from build123d import *

# Parameters (mm, degrees)
BOSS_EXTRUDE1_DEPTH      = 2
BOSS_EXTRUDE1_DEPTH_BACK = 1.043576075
SKETCH1_W                = 32
SKETCH1_H                = 40
CUT_EXTRUDE3_DEPTH       = 26.792699652
CUT_EXTRUDE3_DEPTH_BACK  = 26.792699652
SKETCH5_R                = 1.5
SKETCH5_R_2              = 1
SKETCH_4_W               = 14
SKETCH_4_H               = 4.843949414
CUT_EXTRUDE_3_DEPTH      = 26.792699652
SKETCH_5_W               = 9
SKETCH_5_H               = 3
EXTRUDE_3_DEPTH          = 10
SKETCH_6_R               = 1.5
CUT_EXTRUDE_5_DEPTH      = 44.8178046


with BuildPart() as part:
    # Sketch1 → Boss-Extrude1 (new, two sides: drawn at the far end of the back side and taken through both)
    with BuildSketch(Plane.XY.offset(-BOSS_EXTRUDE1_DEPTH_BACK)):
        Rectangle(SKETCH1_W, SKETCH1_H)
    extrude(amount=BOSS_EXTRUDE1_DEPTH + BOSS_EXTRUDE1_DEPTH_BACK)

    # Sketch5 → Cut-Extrude3 (cut, two sides: drawn at the far end of the back side and taken through both)
    with BuildSketch(Plane.XY.offset(2).offset(-CUT_EXTRUDE3_DEPTH_BACK)):
        Circle(SKETCH5_R)
        with Locations((0, 7.2)):
            Circle(SKETCH5_R_2)
        with Locations((7.2, 0)):
            Circle(SKETCH5_R_2)
        with Locations((0, -7.2)):
            Circle(SKETCH5_R_2)
        with Locations((-7.2, 0)):
            Circle(SKETCH5_R_2)
    extrude(amount=CUT_EXTRUDE3_DEPTH + CUT_EXTRUDE3_DEPTH_BACK, mode=Mode.SUBTRACT)

    # 草图4 → 切除-拉伸3 (cut, through all)
    with BuildSketch(Plane.XY.offset(2)):
        with Locations((0, 17.578025293)):
            Rectangle(SKETCH_4_W, SKETCH_4_H)
        with Locations((0, -17.578025293)):
            Rectangle(SKETCH_4_W, SKETCH_4_H)
    extrude(amount=-CUT_EXTRUDE_3_DEPTH, mode=Mode.SUBTRACT)

    # 草图5 → 凸台-拉伸3 (add)
    with BuildSketch(Plane.XY.offset(2)):
        with Locations((11.5, 18.5)):
            Rectangle(SKETCH_5_W, SKETCH_5_H)
        with Locations((-11.5, 18.5)):
            Rectangle(SKETCH_5_W, SKETCH_5_H)
        with Locations((-11.5, -18.5)):
            Rectangle(SKETCH_5_W, SKETCH_5_H)
        with Locations((11.5, -18.5)):
            Rectangle(SKETCH_5_W, SKETCH_5_H)
    extrude(amount=-EXTRUDE_3_DEPTH)

    # 草图6 → 切除-拉伸5 (cut, through all)
    with BuildSketch(Plane.XZ.offset(20)):
        with Locations(Location((11.6894988, -5, 0), (0, 0, 270))):
            Circle(SKETCH_6_R)
        with Locations(Location((-11.6894988, -5, 0), (0, 0, 270))):
            Circle(SKETCH_6_R)
    extrude(amount=-CUT_EXTRUDE_5_DEPTH, mode=Mode.SUBTRACT)


solid = part.part
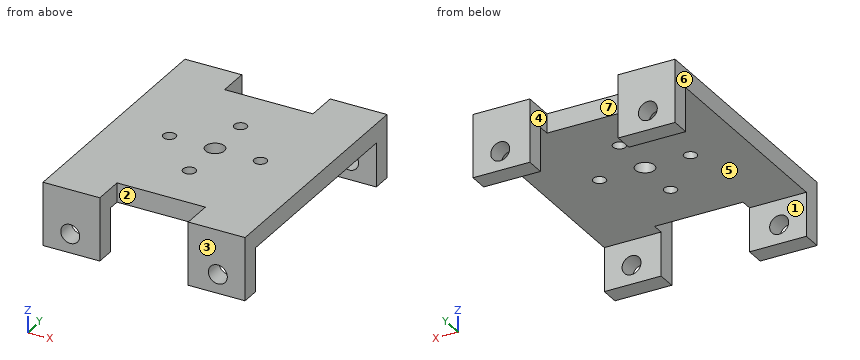
Geometry: final body of the model. Coordinates: model frame, mm. Face numbers are marked on the shaded views. A direction names the side the tool comes from. Coordinates: 2 decimals unless noted, no trailing zeros. Order: outer loops, then holes, each group sorted by start corner. A loop starts at its lowest first (then second) coordinate and runs counter-clockwise, first axis right, second up. Notation, with made-up numbers: M -37,84.25 L -11,84.25 A17 ccw -11,108.25 Z; hole C 69,31.25 d9. An arc over 180 degrees is marked long. One line per question, with ' | ' between items. Start each with the question number.
Item 1: Cut plane C-C, the plane x = 0. Return the cut outline in (y, z), then the cut area to 3 significant figures.
Item 2: Set-up query: the marked faces 1, 2, 3 and 4. Return all of +Z, -Z, +X, -X, +Y, -Y with unobstructed straight access to the full face (end or side cutting, diameter ignored); none if empty.
Item 3: Draft query along Y for the marked faces 5, 6 and 7. Return one class per face: released by +Y, released by -Y, zero draft, split by the parting line, or undercut.
Item 4: Cut plane A-A, the plane y = -7.2. Return the cut outline in (x, z), then the cut area to 3 significant figures.
Item 5: Ray query, probe 1 along X at (y, z) = (18.15, -5); probe 2 along X at (y, z) = (0, 0.4); probe 3 along X at (y, z) = (-7.2, 0.8). Return the intervals inside material, ascending. Write a range as [from, to].
Item 6: Pin query (flat end, axial travel): pin 1 Ø2.5 at (x, y) = (-7.2, 0) entering from -Z; pin 2 Ø2.5 at (x, z) = (-3, 0.5) entering from +Y. Return the tip coordinate at first contact, or that it passes through.
Item 7: Cut plane B-B, the plane z = 0.25. Return the cut outline in (x, y), then the cut area to 3 significant figures.
Item 8: Cut plane D-D, the plane z = -5. Count the separate pieces of the cut face and the enclosed holes in it, then the cut area to 3 significant figures.
A:
1) outline: M -15.16,-1.04 L -8.2,-1.04 L -8.2,2 L -15.16,2 Z; M -6.2,-1.04 L -1.5,-1.04 L -1.5,2 L -6.2,2 Z; M 1.5,-1.04 L 6.2,-1.04 L 6.2,2 L 1.5,2 Z; M 8.2,-1.04 L 15.16,-1.04 L 15.16,2 L 8.2,2 Z | area: 71.0 mm2
2) face 1: -Z, +X, -X | face 2: +Z, -Z, -Y | face 3: +Z, -Z, +X, -X, -Y | face 4: +Z, -Z, +Y
3) face 5: undercut | face 6: zero draft | face 7: released by +Y
4) outline: M -16,-1.04 L -1,-1.04 L -1,2 L -16,2 Z; M 1,-1.04 L 16,-1.04 L 16,2 L 1,2 Z | area: 91.3 mm2
5) probe 1: x = [-16, -13.19], [-10.19, -7], [7, 10.19], [13.19, 16] | probe 2: x = [-16, -8.2], [-6.2, -1.5], [1.5, 6.2], [8.2, 16] | probe 3: x = [-16, -1], [1, 16]
6) pin 1: stops at z = -1.04 | pin 2: stops at y = 15.16
7) outline: M -16,-20 L -7,-20 L -7,-15.16 L 7,-15.16 L 7,-20 L 16,-20 L 16,20 L 7,20 L 7,15.16 L -7,15.16 L -7,20 L -16,20 Z; hole C -7.2,0 d2; hole C 0,0 d3; hole C 0,-7.2 d2; hole C 0,7.2 d2; hole C 7.2,0 d2 | area: 1,120 mm2
8) separate pieces: 8 | enclosed holes: 0 | area: 72.0 mm2
